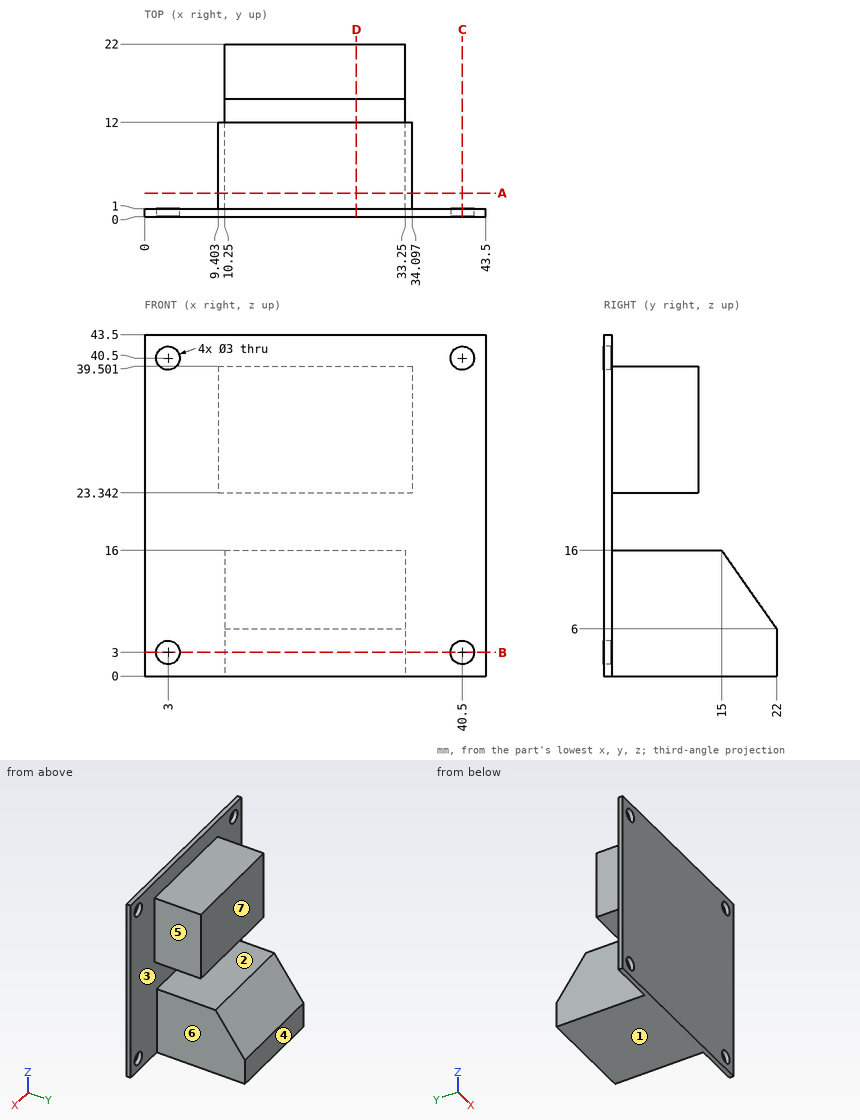
Drawing for the job (mm, zero at the part's lowest x, y, z). A direction names the side the tool comes from. Round coordinates to 2 decimals unless told otherwise and drop trailing zeros. Loops run counter-clockwise (first coordinate to the right, second up) from the corner with the lowest first, then second, coordinate; pieces in that order, holes last. Notation, with made-up numbers: (-36.75, 72.25) -> (-26.75, 72.25) arc R32 cw to (-26.75, 98.25) -> close; hole circle Ø4 at (33, 54). An arc over 180 degrees is marked (long way). Use one line per item in the form item = value. Start each with the question number.
Item 1: Drill centre lines: line 1 along Z through (x, y) = (3, 0.55); line 2 along Z through (x, y) = (28, 5.5). Where is each one in solid material? Low to high.
Item 2: Band-saw the part on D-D (x = 27). List the corners of the cut face in (y, z).
Item 3: Band-saw the part on C-C (x = 40.5). List the corners of the cut face in (y, z).
Item 4: Two-plate mould, pull along Z, no slides. Class the marked faces 1, 2, 3 and 4: released by +Z, released by -Z, zero draft, split by the parting line, or undercut.
Item 5: Drop flat-ended pins along their axis: pin 1 Ø13 at (y, z) = (14, 11) entering from -X; pin 2 Ø8 at (y, z) = (11.5, 6) entering from +X; pin 3 Ø13 at (x, z) = (27.5, 15.5) entering from +Y; pin 4 Ø2.5 at (x, z) = (40.5, 3) entering from -Y. Give the stop position or say it passes through.
Item 6: Tool access for the marked faces 5, 6 and 7: list every direction of +Z, -Z, +X, -X, +Y, -Y with a clear straight run to the whole face (end or side of a thin tool).
Item 7: Band-saw the part on B-B (z = 3). List the corners of the cut face in (x, y).
Item 8: Band-saw the part on A-A (y = 3). List the corners of the cut face in (x, z), plus the area to 3 significant figures.
Data:
q1.line_1 = 0 to 1.5, 4.5 to 39, 42 to 43.5
q1.line_2 = 0 to 16, 23.34 to 39.5
q2.outline = (0, 0) -> (22, 0) -> (22, 6) -> (15, 16) -> (1, 16) -> (1, 23.34) -> (12, 23.34) -> (12, 39.5) -> (1, 39.5) -> (1, 43.5) -> (0, 43.5) -> close
q3.outline = (0, 0) -> (1, 0) -> (1, 1.5) -> (0, 1.5) -> close; (0, 4.5) -> (1, 4.5) -> (1, 39) -> (0, 39) -> close; (0, 42) -> (1, 42) -> (1, 43.5) -> (0, 43.5) -> close
q4.face_1 = released by -Z
q4.face_2 = undercut
q4.face_3 = undercut
q4.face_4 = zero draft
q5.pin_1 = 10.25
q5.pin_2 = 33.25
q5.pin_3 = 19.9
q5.pin_4 = through
q6.face_5 = +Z, -Z, +X, +Y
q6.face_6 = -Z, +X, +Y
q6.face_7 = +Z, +X, -X, +Y
q7.outline = (0, 0) -> (1.5, 0) -> (1.5, 1) -> (0, 1) -> close; (4.5, 0) -> (39, 0) -> (39, 1) -> (33.25, 1) -> (33.25, 22) -> (10.25, 22) -> (10.25, 1) -> (4.5, 1) -> close; (42, 0) -> (43.5, 0) -> (43.5, 1) -> (42, 1) -> close
q8.outline = (9.4, 23.34) -> (34.1, 23.34) -> (34.1, 39.5) -> (9.4, 39.5) -> close; (10.25, 0) -> (33.25, 0) -> (33.25, 16) -> (10.25, 16) -> close
q8.area = 767 mm^2
